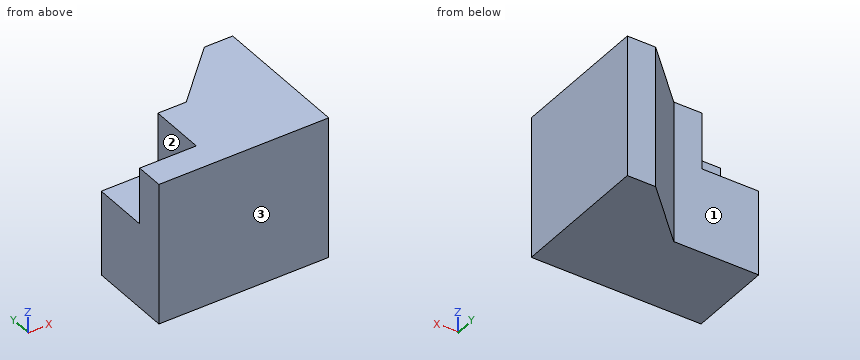
from build123d import *

# Parameters (mm, degrees)
BOSS_EXTRUDE2_DEPTH = 50
SKETCH3_W           = 20
SKETCH3_H           = 20
CUT_EXTRUDE2_DEPTH  = 20


with BuildPart() as part:
    # Sketch1 → Boss-Extrude2 (new body)
    with BuildSketch(Plane.XY):
        Polygon((0, 0), (0, 30), (30, 30), (50, 50), (60, 50), (60, 0), align=None)
    extrude(amount=BOSS_EXTRUDE2_DEPTH)

    # Sketch3 → Cut-Extrude2 (cut)
    with BuildSketch(Plane.XY.offset(50)):
        with Locations((10, 20)):
            Rectangle(SKETCH3_W, SKETCH3_H)
    extrude(amount=-CUT_EXTRUDE2_DEPTH, mode=Mode.SUBTRACT)


solid = part.part
Can you work these out from the model? Positions are in its coordinate system, mm. Face numbers are marked on the shaded views. A direction names the side the tool comes from. Round coordinates to 2 decimals unless told otherwise and drop trailing zeros. Write each loop counter-clockwise with the first axis right and the second up, starting at its lowest first coordinate (ties: lowest second). Pieces come first, ordered by that corner, then holes. Notation, with made-up numbers: (-28, 42) - (2, 42) arc R18 ccw to (2, 56) - close; hole circle Ø10 at (-37, -1.5). An arc over 180 degrees is marked (long way). Write each question's results on one line, items separated by ' | '. Start each with the question number.
1) Suppose I cut it at B-B (x = 18). List the corners of the cut face in (y, z) for me, and give its area (3 significant figures).
2) Suppose I cut it at C-C (y = 26). List the corners of the cut face in (x, z) for me, and give its area (3 significant figures).
3) Suppose I cut it at A-A (z = 34.5). List the corners of the cut face in (x, y) for me, and give its area (3 significant figures).
4) Suppose I cut it at D-D (y = 31.5). List the corners of the cut face in (x, z) for me.
5) Please list where these lines run through material, in increasing order: line 1 (Y direction, x = 7, z = 39); line 2 (Z direction, x = 5, y = 29).
6) For pin 1 Ø6 at (y, z) = (17, 43.5) entering from -X; pin 2 Ø8 at (x, z) = (33, 35.5) entering from +Y; pin 3 Ø1.5 at (x, z) = (49, 35.5) entering from +Y, each with a flat end and sliding along its axis, tell me the tip position at first contact or that it passes through.
7) Which directions (+Z, -Z, +X, -X, +Y, -Y) give clear straight access to the entire face, cutting with the end or side of a thin tool? Please do the marked faces 1, 2 and 3.
Here are the results:
1) outline: (0, 0) - (30, 0) - (30, 30) - (10, 30) - (10, 50) - (0, 50) - close | area: 1,100 mm2
2) outline: (0, 0) - (60, 0) - (60, 50) - (20, 50) - (20, 30) - (0, 30) - close | area: 2,600 mm2
3) outline: (0, 0) - (60, 0) - (60, 50) - (50, 50) - (30, 30) - (20, 30) - (20, 10) - (0, 10) - close | area: 1,800 mm2
4) outline: (31.5, 0) - (60, 0) - (60, 50) - (31.5, 50) - close
5) line 1: y = 0 to 10 | line 2: z = 0 to 30
6) pin 1: stops at x = 20 | pin 2: stops at y = 37 | pin 3: stops at y = 49.75
7) face 1: +Z, -Z, -X, +Y | face 2: +Z, -X, +Y | face 3: +Z, -Z, +X, -X, -Y
